Geometry check sheet. Reference: the model listing, model coordinates, mm. Coordinates: 2 decimals unless noted, no trailing zeros. Loops run counter-clockwise (first coordinate to the right, second up) from the corner with the lowest first, then second, coordinate; pieces in that order, holes last.
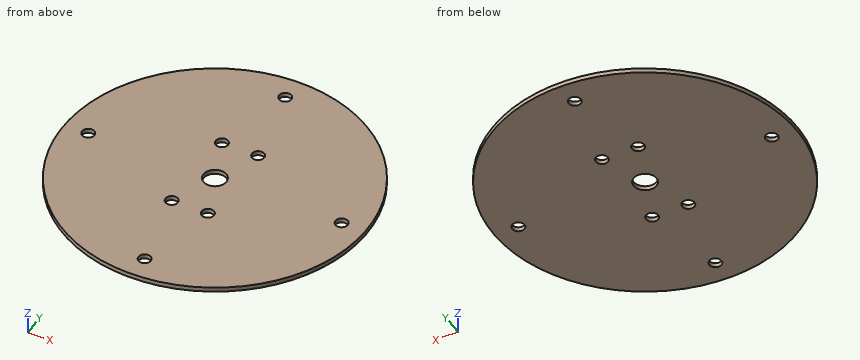
from build123d import *

# Parameters (mm, degrees)
SKETCH1_R           = 84.455
BOSS_EXTRUDE1_DEPTH = 2.54
SKETCH2_R           = 3.429
CUT_EXTRUDE1_DEPTH  = 2.54
SKETCH3_R           = 6.35
CUT_EXTRUDE2_DEPTH  = 2.54
SKETCH4_R           = 3.429
CUT_EXTRUDE3_DEPTH  = 120.464411646
CIRPATTERN1_COUNT   = 4


with BuildPart() as part:
    # Sketch1 → Boss-Extrude1 (new body)
    with BuildSketch(Plane.XY):
        Circle(SKETCH1_R)
    extrude(amount=BOSS_EXTRUDE1_DEPTH)

    # Sketch2 → Cut-Extrude1 (cut)
    with BuildSketch(Plane.XY.offset(2.54)):
        with Locations((-10.16, 25.4)):
            Circle(SKETCH2_R)
        with Locations(Location((10.16, 25.4, 0), (0, 0, 180))):
            Circle(SKETCH2_R)
        with Locations((10.16, -25.4)):
            Circle(SKETCH2_R)
        with Locations(Location((-10.16, -25.4, 0), (0, 0, 180))):
            Circle(SKETCH2_R)
    extrude(amount=-CUT_EXTRUDE1_DEPTH, mode=Mode.SUBTRACT)

    # Sketch3 → Cut-Extrude2 (cut)
    with BuildSketch(Plane.XY.offset(2.54)):
        Circle(SKETCH3_R)
    extrude(amount=-CUT_EXTRUDE2_DEPTH, mode=Mode.SUBTRACT)

    # Sketch4 → Cut-Extrude3 (cut, through all)
    with BuildSketch(Plane(origin=(0, 0, 0), x_dir=(-1, 0, 0), z_dir=(0, 0, -1))):
        with Locations((71.12, 0)):
            Circle(SKETCH4_R)
    cut_extrude3 = extrude(amount=-CUT_EXTRUDE3_DEPTH, mode=Mode.SUBTRACT)

    # CirPattern1: Cut-Extrude3 ×4 about axis
    cirpattern1_axis = Axis((0, 0, 0), (0, 0, 1))
    for i in range(1, CIRPATTERN1_COUNT):
        add(cut_extrude3.rotate(cirpattern1_axis, i * 360 / CIRPATTERN1_COUNT), mode=Mode.SUBTRACT)


solid = part.part
(1) Scan lines: L1, parallel to X at y = -24.5, z = 0.35; L2, parallel to X at y = 27, z = 1.5; L3, parallel to Y at x = -10.16, z = 1.9. Record each from-to range of solid material in increasing order.
Findings:
L1: x = -80.82 to -13.47, -6.85 to 6.85, 13.47 to 80.82
L2: x = -80.02 to -13.19, -7.13 to 7.13, 13.19 to 80.02
L3: y = -83.84 to -28.83, -21.97 to 21.97, 28.83 to 83.84
(2) Sectioned sample at B-B on y = 25.4. Record the cut outline in (x, z).
Findings:
outline: (-80.54, 0) - (-13.59, 0) - (-13.59, 2.54) - (-80.54, 2.54) - close; (-6.73, 0) - (6.73, 0) - (6.73, 2.54) - (-6.73, 2.54) - close; (13.59, 0) - (80.54, 0) - (80.54, 2.54) - (13.59, 2.54) - close
(3) Sectioned sample at D-D on x = -71.12. Record the cut outline in (y, z), and give its area (3 significant figures).
Findings:
outline: (-45.55, 0) - (-3.43, 0) - (-3.43, 2.54) - (-45.55, 2.54) - close; (3.43, 0) - (45.55, 0) - (45.55, 2.54) - (3.43, 2.54) - close
area: 214 mm2
(4) Gauge pin test, flat end, axial feed: pin 1 Ø9 at (x, y) = (10.16, -25.4) entering from -Z. Record the tip position at first contact, or that the pin passes through.
Findings:
pin 1: stops at z = 0
(5) Sectioned sample at C-C on z = 1.35. State how many separate pieces and enclosed holes the cut face has, and give its area (3 significant figures).
Findings:
separate pieces: 1
enclosed holes: 9
area: 22,000 mm2
(6) Sectioned sample at A-A on x = 0. Record the cut outline in (y, z) (3 decimals).
Findings:
outline: (-84.455, 0) - (-74.549, 0) - (-74.549, 2.54) - (-84.455, 2.54) - close; (-67.691, 0) - (-6.35, 0) - (-6.35, 2.54) - (-67.691, 2.54) - close; (6.35, 0) - (67.691, 0) - (67.691, 2.54) - (6.35, 2.54) - close; (74.549, 0) - (84.455, 0) - (84.455, 2.54) - (74.549, 2.54) - close
